Study the drawing (mm; zero at the part's minimum x, y, z) and answer. Give positions to 0.01 mm unless a question says otherwise; leave off trailing zeros. Order: outer loops, then holes, each group sorted by start corner. A loop starts at its lowest first (then second) coordinate and runs counter-clockwise, first axis right, second up.
Item 1: Find the intervals of material crossed by line 1 along X through (y, z) = (0.8, 28.5); line 2 along Z through (x, y) = (5.5, 0.55); line 3 along X through (y, z) = (1.15, 28.5), in increasing order.
Item 2: A cutting plane is placed at C-C (x = 5.5). Write down the section's boundary in (y, z), plus the area to 3 significant figures.
Item 3: A cutting plane is placed at A-A (x = 27). State how many separate pieces and enclosed holes the cut face has.
Item 4: A cutting plane is placed at D-D (z = 7). Write down the section's boundary in (x, y).
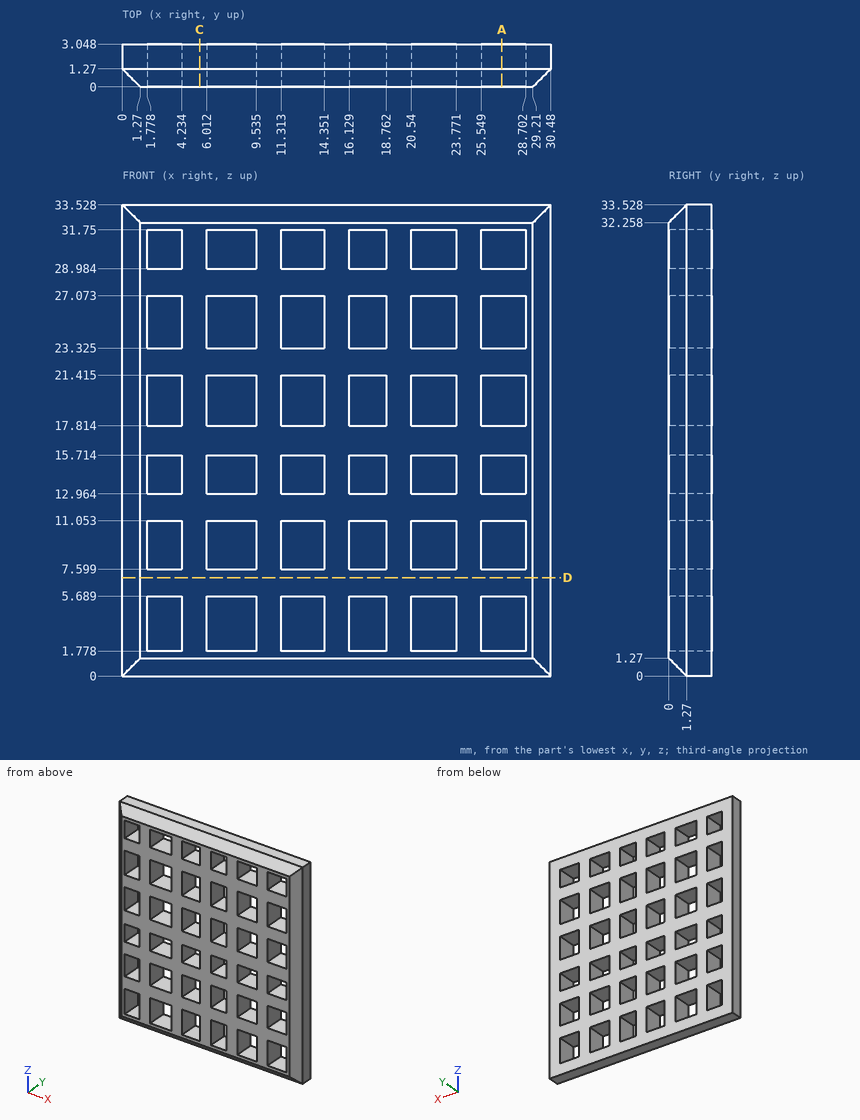
Response values:
1. line 1: x = 0.47 to 30.01
1. line 2: z = 0.72 to 32.81
1. line 3: x = 0.12 to 30.36
2. outline: (0, 1.27) - (1.27, 0) - (3.05, 0) - (3.05, 33.53) - (1.27, 33.53) - (0, 32.26) - close
2. area: 101 mm2
3. separate pieces: 7
3. enclosed holes: 0
4. outline: (0, 1.27) - (1.27, 0) - (29.21, 0) - (30.48, 1.27) - (30.48, 3.05) - (0, 3.05) - close
